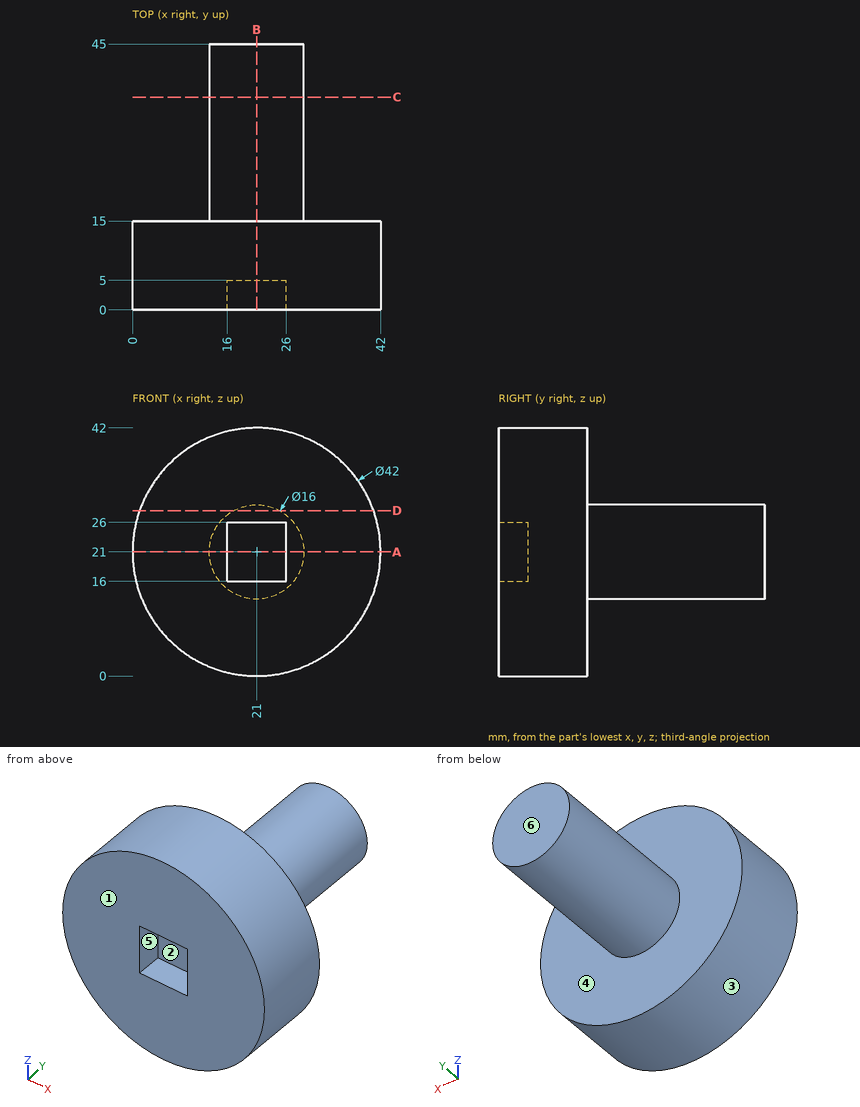
Check sheet for the drawn part. Datum: minimum x, y, z corner. Units: mm. A direction names the side the tool comes from. Coordinates: 2 decimals unless noted, no trailing zeros. Order: outer loops, then holes, each group sorted by start corner. A loop starts at its lowest first (then second) coordinate and runs counter-clockwise, first axis right, second up. Notation, with made-up numbers: M -19,69 L 27,69 A12 cw 27,87 Z; hole C 58,23 d5. An arc over 180 degrees is marked long. One line per item, written item: value. Start each with the question number.
Item 1: Sectioned sample at A-A (z = 21). Enter the section's corners in (x, y).
Item 2: Sectioned sample at D-D (z = 28). Enter the section's corners in (x, y).
Item 3: Sectioned sample at B-B (x = 21). Enter the section's corners in (y, z), then the cut area to 3 significant figures.
Item 4: Sectioned sample at C-C (y = 36). Enter the section's corners in (x, z), then the cut area to 3 significant figures.
Item 5: Scan lines: probe 1 along Y at (x, z) = (28.5, 15.5); probe 2 along Y at (x, z) = (17.5, 19); probe 3 along X at (y, z) = (10.5, 30). Record each from-to range of solid material in increasing order.
Item 6: Mould release check, pull along X, two halves, no side actions. Record for the marked faces 1, 2 and 3: released by +X, released by -X, zero draft, split by the parting line, or undercut.
Item 7: Gauge pin test, flat ends, axial feed: pin 1 (1.5 mm diameter, centred on x = 16, z = 33.5, fed in from +Y); pin 2 (5.5 mm diameter, centred on x = 19.5, y = 3.5, fed in from -Z); pin 3 (1.5 mm diameter, centred on x = 22, y = 2, fed in from +Z). Record the tip position at first contact, or that the pin passes through.
Item 8: Access from +Z, -Z, +X, -X, +Y, -Y to the whole of each face (thin tool, end or side, straight path). Record for the marked faces 4, 5 and 6.
Conclusion:
1. outline: M 0,0 L 16,0 L 16,5 L 26,5 L 26,0 L 42,0 L 42,15 L 29,15 L 29,45 L 13,45 L 13,15 L 0,15 Z
2. outline: M 1.2,0 L 40.8,0 L 40.8,15 L 24.87,15 L 24.87,45 L 17.13,45 L 17.13,15 L 1.2,15 Z
3. outline: M 0,0 L 15,0 L 15,13 L 45,13 L 45,29 L 15,29 L 15,42 L 0,42 L 0,26 L 5,26 L 5,16 L 0,16 Z
3. area: 1,060 mm^2
4. outline: C 21,21 d16
4. area: 201 mm^2
5. probe 1: y = 0 to 15
5. probe 2: y = 5 to 45
5. probe 3: x = 2.03 to 39.97
6. face 1: zero draft
6. face 2: undercut
6. face 3: split by the parting line
7. pin 1: stops at y = 15
7. pin 2: stops at z = 0
7. pin 3: stops at z = 42
8. face 4: +Y
8. face 5: -Y
8. face 6: +Z, -Z, +X, -X, +Y
